For this review, take the finished solid that the model builds, in its own axes (mm). A direction names the side the tool comes from. Give positions to 0.01 mm unless a question says otherwise; leave off trailing zeros. Order: outer loops, then holes, each group sorted by start corner. A loop starts at its lowest first (then second) coordinate and runs counter-clockwise, first axis right, second up.
Item 1: Consider section B-B (y = 25). Give the boundary of the cut face in (x, z), plus the area to 3 significant figures.
Item 2: Machinability: for faces 1 (the flat face through (5, 5, 1)), 2 (the flat face through (20, 30, 5)), which of the approach directions +Z, -Z, +X, -X, +Y, -Y give a long, thin tool a straight path to every point of the face, cutting with its end or side? Answer none if there is none.
Item 3: Consider section A-A (z = 5). Give the number of separate pieces and of enclosed holes in the cut face, plus the area to 3 significant figures.
Item 4: For probe 1 along X at (y, z) = (44, 7.5); probe 2 along X at (y, z) = (14, 3.5); probe 3 along Z at (x, y) = (17.5, 42.5), list the stretches that pass through material, from the lowest coordinate up.
Item 5: For P1, Ø0.6, axis at x = 15, y = 15, coming from the +Z side; P2, Ø5, axis at x = 10, y = 47.5, coming from the -Z side, all flat-tipped, find the tip position at first contact; note any pin that passes through.
Item 6: The part is to be moulded in two halves that separate along Y. For faces 3 (the conical face through (3.48, 6.4, 4.56)), 4 (the flat face through (10, 0, 5)), 5 (the flat face through (10, 31, 10)), say which applies: released by +Y, released by -Y, zero draft, split by the parting line, or undercut.
```python
from build123d import *

# Parameters (mm, degrees)
ARRAY_X_COUNT = 2
ARRAY_X_PITCH = 10
ARRAY_Y_COUNT = 6
ARRAY_Y_PITCH = 10
BOX_W         = 20
BOX_H         = 60
BOX_DEPTH     = 10
CHAMFER_SIZE  = 0.5


with BuildPart() as array:
    # Cone → Cone (revolve)
    with BuildSketch(Plane(origin=(5, 5, 1), x_dir=(1, 0, 0), z_dir=(0, -1, 0))):
        Polygon((0, 0), (1, 0), (4, 10), (0, 10), align=None)
    revolve(axis=Axis((5, 5, 1), (0, 0, 1)))

    # Array X: Array ×2


with BuildPart() as array_1:
    add(array.part)
    with Locations(*[(i * ARRAY_X_PITCH, 0, 0) for i in range(1, ARRAY_X_COUNT)]):
        add(array.part)

    # Array Y: Array ×6


with BuildPart() as array_2:
    add(array_1.part)
    with Locations(*[(0, i * ARRAY_Y_PITCH, 0) for i in range(1, ARRAY_Y_COUNT)]):
        add(array_1.part)


with BuildPart() as chamfer_body:
    # Box → Box (new body)
    with BuildSketch(Plane.XY):
        with Locations((10, 30)):
            Rectangle(BOX_W, BOX_H)
    extrude(amount=BOX_DEPTH)

    # Cut: cut Array
    add(array_2.part, mode=Mode.SUBTRACT)

    # Chamfer
    chamfer_edges = [chamfer_body.edges().sort_by_distance(p)[0] for p in [
        (20, 0, 5),
        (10, 0, 10),
        (20, 30, 10),
    ]]
    chamfer(chamfer_edges, length=CHAMFER_SIZE)


solid = chamfer_body.part
```
Resolved:
1. outline: (0, 0) - (20, 0) - (20, 9.5) - (19.5, 10) - (18.7, 10) - (16, 1) - (14, 1) - (11.3, 10) - (8.7, 10) - (6, 1) - (4, 1) - (1.3, 10) - (0, 10) - close
1. area: 115 mm2
2. face 1: +Z
2. face 2: +Z, -Z, +X, +Y, -Y
3. separate pieces: 1
3. enclosed holes: 12
3. area: 1,020 mm2
4. probe 1: x = 0 to 2.22, 7.78 to 12.22, 17.78 to 20
4. probe 2: x = 0 to 3.56, 6.44 to 13.56, 16.44 to 20
4. probe 3: z = 0 to 9.45
5. P1: stops at z = 1
5. P2: stops at z = 0
6. face 3: undercut
6. face 4: released by -Y
6. face 5: zero draft
